```python
from build123d import *

# Parameters (mm, degrees)
SKETCH1_R           = 7.0612
SKETCH1_R_2         = 5.0165
BOSS_EXTRUDE1_DEPTH = 15.24
SKETCH2_R           = 12.66825
SKETCH2_R_2         = 7.0612
BOSS_EXTRUDE2_DEPTH = 7.62
SKETCH3_R           = 14.2494
SKETCH3_R_2         = 12.66825
BOSS_EXTRUDE3_DEPTH = 7.112
SKETCH4_R           = 16.8275
SKETCH4_R_2         = 14.2494
BOSS_EXTRUDE4_DEPTH = 9.398
SKETCH5_R           = 16.8275
BOSS_EXTRUDE5_DEPTH = 5.842
CUT_EXTRUDE1_REACH  = 39.194
SKETCH6_R           = 3.6195


with BuildPart() as part:
    # Sketch1 → Boss-Extrude1 (new body)
    with BuildSketch(Plane(origin=(0, 0, 0), x_dir=(1, 0, 0), z_dir=(0, 1, 0))):
        with Locations(Location((0, 0, 0), (0, 0, 90))):
            Circle(SKETCH1_R)
        with Locations(Location((0, 0, 0), (0, 0, 90))):
            Circle(SKETCH1_R_2, mode=Mode.SUBTRACT)
    extrude(amount=BOSS_EXTRUDE1_DEPTH)

    # Sketch2 → Boss-Extrude2 (add)
    with BuildSketch(Plane(origin=(0, 0, 0), x_dir=(1, 0, 0), z_dir=(0, 1, 0))):
        with Locations(Location((0, 0, 0), (0, 0, 90))):
            Circle(SKETCH2_R)
        with Locations(Location((0, 0, 0), (0, 0, 90))):
            Circle(SKETCH2_R_2, mode=Mode.SUBTRACT)
    extrude(amount=BOSS_EXTRUDE2_DEPTH)

    # Sketch3 → Boss-Extrude3 (add)
    with BuildSketch(Plane.XZ):
        with Locations(Location((0, 0, 0), (0, 0, 270))):
            Circle(SKETCH3_R)
        with Locations(Location((0, 0, 0), (0, 0, 270))):
            Circle(SKETCH3_R_2, mode=Mode.SUBTRACT)
    extrude(amount=-BOSS_EXTRUDE3_DEPTH)

    # Sketch4 → Boss-Extrude4 (add)
    with BuildSketch(Plane.XZ):
        with Locations(Location((0, 0, 0), (0, 0, 270))):
            Circle(SKETCH4_R)
        with Locations(Location((0, 0, 0), (0, 0, 270))):
            Circle(SKETCH4_R_2, mode=Mode.SUBTRACT)
    extrude(amount=-BOSS_EXTRUDE4_DEPTH)

    # Sketch5 → Boss-Extrude5 (add)
    with BuildSketch(Plane(origin=(0, 0, 0), x_dir=(1, 0, 0), z_dir=(0, 1, 0))):
        with BuildLine():
            ThreePointArc((-11.43, 13.867010141), (-17.9705, 0), (-11.43, -13.867010141))
            Line((-11.43, -13.867010141), (-5.419746982, -29.547574395))
            ThreePointArc((-5.419746982, -29.547574395), (-4.487192662, -30.731422474), (-3.048, -31.1785))
            Line((-3.048, -31.1785), (3.048, -31.1785))
            ThreePointArc((3.048, -31.1785), (4.487192662, -30.731422474), (5.419746982, -29.547574395))
            Line((5.419746982, -29.547574395), (11.43, -13.867010141))
            ThreePointArc((11.43, -13.867010141), (17.9705, 0), (11.43, 13.867010141))
            Line((11.43, 13.867010141), (5.419746982, 29.547574395))
            ThreePointArc((5.419746982, 29.547574395), (4.487192662, 30.731422474), (3.048, 31.1785))
            Line((3.048, 31.1785), (-3.048, 31.1785))
            ThreePointArc((-3.048, 31.1785), (-4.487192662, 30.731422474), (-5.419746982, 29.547574395))
            Line((-5.419746982, 29.547574395), (-11.43, 13.867010141))
        make_face()
        with Locations(Location((0, 0, 0), (0, 0, 90))):
            Circle(SKETCH5_R, mode=Mode.SUBTRACT)
    extrude(amount=BOSS_EXTRUDE5_DEPTH)

    # Sketch6 → Cut-Extrude1 (cut, up to next)
    with BuildSketch(Plane(origin=(0, 5.842, 0), x_dir=(1, 0, 0), z_dir=(0, 1, 0)), mode=Mode.PRIVATE) as cut_extrude1_sk1:
        with Locations(Location((0, 23.622, 0), (0, 0, 270))):
            Circle(SKETCH6_R)
    cut_extrude1_tool1 = extrude(cut_extrude1_sk1.sketch, amount=-CUT_EXTRUDE1_REACH, mode=Mode.PRIVATE) & part.part
    # Sketch6 → Cut-Extrude1 (cut, up to next)
    with BuildSketch(Plane(origin=(0, 5.842, 0), x_dir=(1, 0, 0), z_dir=(0, 1, 0)), mode=Mode.PRIVATE) as cut_extrude1_sk2:
        with Locations(Location((0, -23.622, 0), (0, 0, 270))):
            Circle(SKETCH6_R)
    cut_extrude1_tool2 = extrude(cut_extrude1_sk2.sketch, amount=-CUT_EXTRUDE1_REACH, mode=Mode.PRIVATE) & part.part
    add(cut_extrude1_tool1.solids().sort_by_distance((0, 5.842, -23.622))[0], mode=Mode.SUBTRACT)
    add(cut_extrude1_tool2.solids().sort_by_distance((0, 5.842, 23.622))[0], mode=Mode.SUBTRACT)


solid = part.part
```
Geometry: final body of the model. Coordinates: model frame, mm. A direction names the side the tool comes from. Coordinates: 2 decimals unless noted, no trailing zeros. Write each loop counter-clockwise with the first axis right and the second up, starting at its lowest first coordinate (ties: lowest second). Pieces come first, ordered by that corner, then holes. Notation, with made-up numbers: M 74,86 L 85,86 A11 cw 85,92 Z; hole C -23.75,75.25 d2. An arc over 180 degrees is marked long. Answer as CSV lines item,"result". Start each with the question number.
Q1. Reachability of faces 1 (the flat face through (11, 5.842, 14)), 2 (the cylindrical face through (-17.97, 2.88, -0.22)) from +Z, -Z, +X, -X, +Y, -Y: full face, straight path, thin tool, end or side. Return the list, or none.
Q2. Cut plane D-D on x = -13.5. Return the cut outline in (y, z), then the cut area to 3 significant figures.
Q3. Pin query (flat end, axial travel): P1, Ø6, axis at y = 6, z = 6.5, coming from the -X side; P2, Ø5, axis at y = 10.5, z = 4.5, coming from the -X side; P3, Ø5, axis at y = 11.5, z = -11.5, coming from the -X side. Return the tip coordinate at first contact, or that it passes through.
Q4. Line query: line 1 (X direction, y = 8, z = 0); line 2 (Z direction, x = 3, y = 1.5); line 3 (Y direction, x = -2.5, z = 11). Output: solid intervals per line, ascending. Write a range as from..to.
Q5. Cut plane A-A on y = 3.75. Return the cut outline in (x, z), then the cut area to 3 significant figures.
Q6. Mould query, pull axis Z, two halves, no side actions, for faces 3 (the flat face through (5.5, 7.62, -5.5)), 4 (the flat face through (8.38, 2.88, 21.82)), 5 (the flat face through (-5, 15.24, 2)). Classes: released by +Z, released by -Z, zero draft, split by the parting line, or undercut.
Q7. Cut plane B-B on x = 0. Count the separate pieces of the cut face and the enclosed holes in it, then the cut area to 3 significant figures.
Q8. Cut plane C-C on z = 0. Return the cut outline in (x, y), then the cut area to 3 significant figures.
Findings below:
1,face 1,"+Y"
1,face 2,"-X, +Y, -Y"
2,outline,"M 0,-11.86 L 5.84,-11.86 L 5.84,-10.05 L 9.4,-10.05 L 9.4,-4.56 L 7.11,-4.56 L 7.11,4.56 L 9.4,4.56 L 9.4,10.05 L 5.84,10.05 L 5.84,11.86 L 0,11.86 Z"
2,area,"189 mm2"
3,P1,"stops at x = -17.63"
3,P2,"stops at x = -16.68"
3,P3,"stops at x = -13.42"
4,line 1,"x = -16.83..-14.25, -7.06..-5.02, 5.02..7.06, 14.25..16.83"
4,line 2,"z = -31.18..-25.65, -21.6..-4.02, 4.02..21.6, 25.65..31.18"
4,line 3,"y = 0..7.62"
5,outline,"M -11.43,-13.87 L -5.42,-29.55 A2.54 ccw -3.05,-31.18 L 3.05,-31.18 A2.54 ccw 5.42,-29.55 L 11.43,-13.87 A17.97 ccw 11.43,13.87 L 5.42,29.55 A2.54 ccw 3.05,31.18 L -3.05,31.18 A2.54 ccw -5.42,29.55 L -11.43,13.87 A17.97 ccw Z; hole C 0,0 d10.03; hole C 0,-23.62 d7.24; hole C 0,23.62 d7.24"
5,area,"1,280 mm2"
6,face 3,"undercut"
6,face 4,"released by +Z"
6,face 5,"zero draft"
7,separate pieces,"4"
7,enclosed holes,"0"
7,area,"302 mm2"
8,outline,"M -17.97,0 L -5.02,0 L -5.02,15.24 L -7.06,15.24 L -7.06,7.62 L -12.67,7.62 L -12.67,7.11 L -14.25,7.11 L -14.25,9.4 L -16.83,9.4 L -16.83,5.84 L -17.97,5.84 Z; M 5.02,0 L 17.97,0 L 17.97,5.84 L 16.83,5.84 L 16.83,9.4 L 14.25,9.4 L 14.25,7.11 L 12.67,7.11 L 12.67,7.62 L 7.06,7.62 L 7.06,15.24 L 5.02,15.24 Z"
8,area,"232 mm2"
